Part print with two shaded views. Sizes in mm from the minimum x, y, z corner. Coordinates: 2 decimals unless noted, no trailing zeros. Loops run counter-clockwise (first coordinate to the right, second up) from the corner with the lowest first, then second, coordinate; pieces in that order, holes last. Notation, with made-up numbers: (10, 63.5) -> (19, 63.5) arc R38 cw to (19, 101.5) -> close; hole circle Ø2 at (44.5, 16). An arc over 180 degrees is marked (long way). One line per item, written item: value. Start each with the question number.
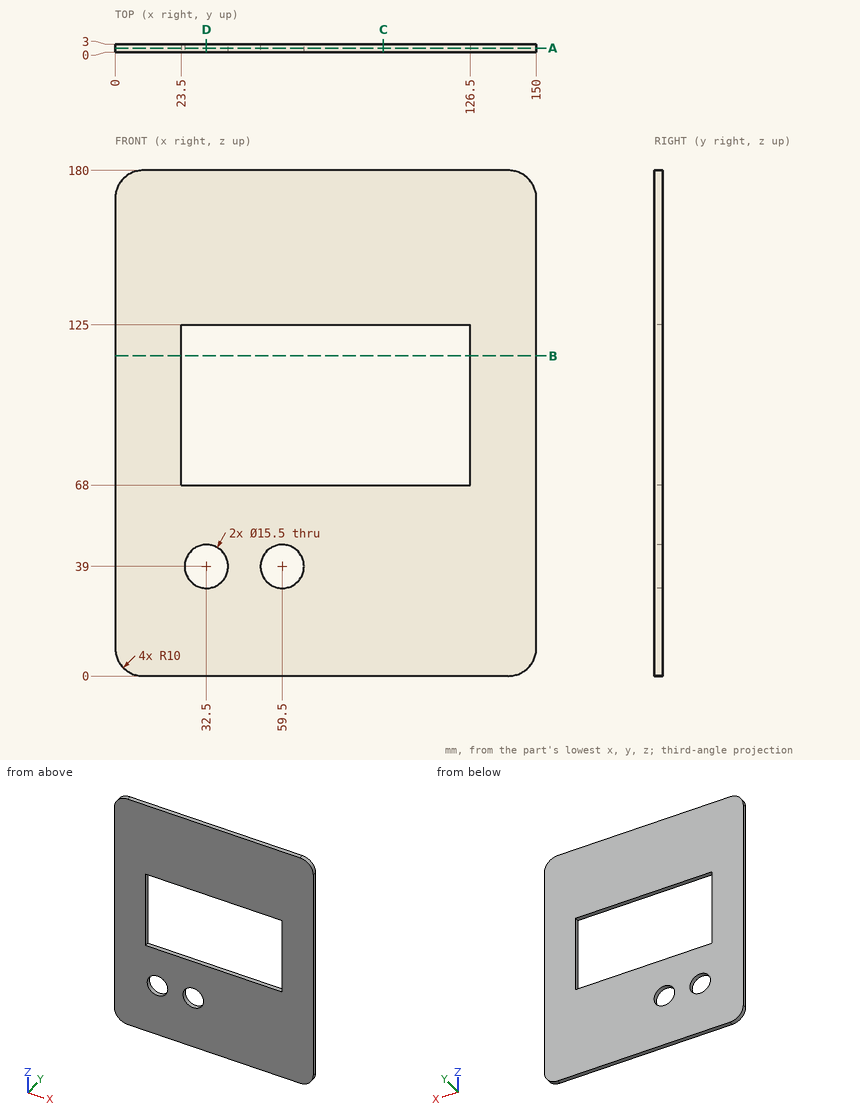
Item 1: Probe probe 1 along Z at (x, y) = (59.5, 1.35); probe 2 along X at (y, z) = (2.4, 87); probe 3 along X at (y, z) = (1.9, 41.5). List the from-to ranges inside material, lowest first.
Item 2: Band-saw the part on A-A, the plane y = 1.55. List the corners of the cut face in (x, z), and give its area (3 significant figures).
Item 3: Band-saw the part on C-C, the plane x = 95.5. List the corners of the cut face in (y, z).
Item 4: Band-saw the part on D-D, the plane x = 32.5. List the corners of the cut face in (y, z).
Item 5: Band-saw the part on B-B, the plane z = 114. List the corners of the cut face in (x, y), and give its area (3 significant figures).
Worked out:
1. probe 1: z = 0 to 31.25, 46.75 to 68, 125 to 180
1. probe 2: x = 0 to 23.5, 126.5 to 150
1. probe 3: x = 0 to 25.16, 39.84 to 52.16, 66.84 to 150
2. outline: (0, 10) arc R10 ccw to (10, 0) -> (140, 0) arc R10 ccw to (150, 10) -> (150, 170) arc R10 ccw to (140, 180) -> (10, 180) arc R10 ccw to (0, 170) -> close; hole (23.5, 68) -> (126.5, 68) -> (126.5, 125) -> (23.5, 125) -> close; hole circle Ø15.5 at (32.5, 39); hole circle Ø15.5 at (59.5, 39)
2. area: 20,700 mm²
3. outline: (0, 0) -> (3, 0) -> (3, 68) -> (0, 68) -> close; (0, 125) -> (3, 125) -> (3, 180) -> (0, 180) -> close
4. outline: (0, 0) -> (3, 0) -> (3, 31.25) -> (0, 31.25) -> close; (0, 46.75) -> (3, 46.75) -> (3, 68) -> (0, 68) -> close; (0, 125) -> (3, 125) -> (3, 180) -> (0, 180) -> close
5. outline: (0, 0) -> (23.5, 0) -> (23.5, 3) -> (0, 3) -> close; (126.5, 0) -> (150, 0) -> (150, 3) -> (126.5, 3) -> close
5. area: 141 mm²
